For this review, take the finished solid that the model builds, in its own axes (mm). A direction names the side the tool comes from. Round coordinates to 2 decimals unless told otherwise and drop trailing zeros. Write each loop counter-clockwise with the first axis right and the second up, starting at its lowest first coordinate (ties: lowest second). Pieces come first, ordered by that corner, then holes. Notation, with made-up numbers: M 69,51.5 L 123,51.5 A31 ccw 123,81.5 Z; hole C -14,24.5 d2. An arc over 180 degrees is marked long. One line per question, with ' | ' between items.
```python
from build123d import *

# Parameters (mm, degrees)
F1_DEPTH  = 18.9992
F2_START  = -41.3258
F2_DEPTH  = 18.9992
F3_DEPTH  = 60.325
F4_DEPTH  = 60.325
F5_START  = -19.05
F5_DEPTH  = 41.275
F6_DEPTH  = 25.4
F7_R      = 3.302
F8_R      = 7.874
F9_R      = 6.35
F10_DEPTH = 22.353


with BuildPart() as f1:
    # F0 (on Front) → F1 (new body)
    with BuildSketch(Plane.XZ):
        with BuildLine():
            ThreePointArc((-171.8564, 22.352), (-210.0136507731, 38.1572507731), (-194.2084, 0))
            Line((-194.2084, 0), (-194.2084, 9.652))
            ThreePointArc((-194.2084, 9.652), (-203.1886561211, 31.3322561211), (-181.5084, 22.352))
            Line((-181.5084, 22.352), (-171.8564, 22.352))
        make_face()
        with BuildLine():
            Line((-194.2084, 9.652), (-194.2084, 0))
            ThreePointArc((-194.2084, 0), (-178.4031492269, 6.5467492269), (-171.8564, 22.352))
            Line((-171.8564, 22.352), (-181.5084, 22.352))
            ThreePointArc((-181.5084, 22.352), (-185.2281438789, 13.3717438789), (-194.2084, 9.652))
        make_face()
        with BuildLine():
            Line((-194.2084, 0), (-149.7584, 0))
            Line((-149.7584, 0), (-166.2684, 22.352))
            Line((-166.2684, 22.352), (-171.8564, 22.352))
            ThreePointArc((-171.8564, 22.352), (-178.4031492269, 6.5467492269), (-194.2084, 0))
        make_face()
        Polygon((-149.7584, 0), (-102.362, 0), (-108.3564, 22.352), (-166.2684, 22.352), align=None)
    extrude(amount=-F1_DEPTH)



with BuildPart() as f2:
    # F0 (on Front) → F2 (new body)
    with BuildSketch(Plane.XZ.offset(F2_START)):
        with BuildLine():
            ThreePointArc((-171.8564, 22.352), (-210.0136507731, 38.1572507731), (-194.2084, 0))
            Line((-194.2084, 0), (-194.2084, 9.652))
            ThreePointArc((-194.2084, 9.652), (-203.1886561211, 31.3322561211), (-181.5084, 22.352))
            Line((-181.5084, 22.352), (-171.8564, 22.352))
        make_face()
        with BuildLine():
            Line((-194.2084, 0), (-149.7584, 0))
            Line((-149.7584, 0), (-166.2684, 22.352))
            Line((-166.2684, 22.352), (-171.8564, 22.352))
            ThreePointArc((-171.8564, 22.352), (-178.4031492269, 6.5467492269), (-194.2084, 0))
        make_face()
        with BuildLine():
            Line((-194.2084, 9.652), (-194.2084, 0))
            ThreePointArc((-194.2084, 0), (-178.4031492269, 6.5467492269), (-171.8564, 22.352))
            Line((-171.8564, 22.352), (-181.5084, 22.352))
            ThreePointArc((-181.5084, 22.352), (-185.2281438789, 13.3717438789), (-194.2084, 9.652))
        make_face()
        Polygon((-149.7584, 0), (-102.362, 0), (-108.3564, 22.352), (-166.2684, 22.352), align=None)
    extrude(amount=-F2_DEPTH)


with BuildPart() as f1_1:
    add(f1.part)

    add(f2.part)  # F3 merges F2
    # F0 (on Front) → F3 (join, through all)
    with BuildSketch(Plane.XZ):
        Polygon((-149.7584, 0), (-102.362, 0), (-108.3564, 22.352), (-166.2684, 22.352), align=None)
    extrude(amount=-F3_DEPTH)



with BuildPart() as f4:
    # F0 (on Front) → F4 (new body)
    with BuildSketch(Plane.XZ):
        Polygon((-76.962, 0), (0, 0), (0, 22.352), (-44.1198, 22.352), (-76.962, 22.352), align=None)
    extrude(amount=-F4_DEPTH)


with BuildPart() as f1_2:
    add(f1_1.part)

    add(f4.part)  # F5 merges F4
    # F0 (on Front) → F5 (join)
    with BuildSketch(Plane.XZ.offset(F5_START)):
        Polygon((-102.362, 0), (-76.962, 0), (-76.962, 22.352), (-108.3564, 22.352), align=None)
    extrude(amount=-F5_DEPTH)

    # F0 (on Front) → F6 (join)
    with BuildSketch(Plane.XZ):
        with BuildLine():
            ThreePointArc((-63.1698, 57.15), (-66.7439846384, 38.4343576341), (-76.962, 22.352))
            Line((-76.962, 22.352), (-44.1198, 22.352))
            Line((-44.1198, 22.352), (-44.1198, 52.07))
            ThreePointArc((-44.1198, 52.07), (-45.6076975516, 55.6621024484), (-49.1998, 57.15))
            Line((-49.1998, 57.15), (-63.1698, 57.15))
        make_face()
    extrude(amount=-F6_DEPTH)

    # F7
    f7_edges = [f1_2.edges().sort_by_distance(p)[0] for p in [
        (-44.1198, 12.7, 22.352),
        (-171.8564, 9.4996, 22.352),
        (-171.8564, 50.8254, 22.352),
    ]]
    fillet(f7_edges, radius=F7_R)

    # F8
    f8_edges = [f1_2.edges().sort_by_distance(p)[0] for p in [
        (0, 30.1625, 22.352),
    ]]
    fillet(f8_edges, radius=F8_R)

    # F9 (on face) → F10 (cut, through all)
    with BuildSketch(Plane.XY.offset(22.352)):
        with Locations((-38.862, 37.973)):
            Circle(F9_R)
    extrude(amount=-F10_DEPTH, mode=Mode.SUBTRACT)


solid = f1_2.part
```
Item 1: Mouldability with a two-part tool opening along Y and no side actions: class faces 5 (the face through (-93, 19.05, 11)), 6 (the face through (-56, 13, 57.15)), 7 (the face through (-158.129, 30.006, 11.332)) as +Y half, -Y half, draft (parallel to the pull), parting line (faces both ways), or undercut.
Results:
face 5: -Y half | face 6: draft | face 7: undercut
Item 2: Take a section at A-A (y = 16). Write out the cut boundary in (x, z), then the cut area to 3 significant figures.
Results:
outline: M -194.21,0 L -102.36,0 L -108.36,22.35 L -168.77,22.35 A3.3 cw -172.04,25.23 A22.35 ccw long Z; M -76.96,0 L 0,0 L 0,14.48 A7.87 ccw -7.87,22.35 L -40.82,22.35 A3.3 cw -44.12,25.65 L -44.12,52.07 A5.08 ccw -49.2,57.15 L -63.17,57.15 A50.8 cw -76.96,22.35 Z; hole C -194.21,22.35 d25.4 | area: 5,180 mm2
Item 3: To check wall thickness, follow line 1 along X through (y, z) = (14.5, 13); line 2 along X through (y, z) = (16, 17.5); line 3 along Y through (x, z) = (-179, 33.5) (3 decimals). State the ranges of each line that lie inside material, in increasing order. Write a range as from..to.
Results:
line 1: -214.51..-202.8, -185.62..-105.85, -76.96..0 | line 2: -216.03..-205.95, -182.47..-107.06, -76.96..-0.6 | line 3: 0..18.999, 41.326..60.325
Item 4: Take a section at B-B (x = -198). Write out the cut boundary in (y, z) (3 decimals).
Results:
outline: M 0,0.324 L 18.999,0.324 L 18.999,10.231 L 0,10.231 Z; M 0,34.473 L 18.999,34.473 L 18.999,44.38 L 0,44.38 Z; M 41.326,0.324 L 60.325,0.324 L 60.325,10.231 L 41.326,10.231 Z; M 41.326,34.473 L 60.325,34.473 L 60.325,44.38 L 41.326,44.38 Z
Item 5: Insertion check: pin 1 Ø5.5 at (y, z) = (5, 7) entering from -X; pin 2 Ø3 at (y, z) = (10.5, 43.5) entering from +X; pin 3 Ø20.5 at (x, z) = (-194.21, 22.35) entering from -Y; pin 4 Ø8 at (y, z) = (49.5, 27.5) entering from +X. Each pin has a flat end and moves straight along its axis. Give the tip position at first contact, or say it passes through.
Results:
pin 1: x = -212.67 | pin 2: x = -44.12 | pin 3: through | pin 4: x = -171.27
Item 6: Take a section at D-D (z = 38). Write out the cut boundary in (x, y) (3 decimals), then the cut area to 3 significant figures.
Results:
outline: M -210.169,0 L -178.247,0 L -178.247,18.999 L -210.169,18.999 Z; M -210.169,41.326 L -178.247,41.326 L -178.247,60.325 L -210.169,60.325 Z; M -66.918,0 L -44.12,0 L -44.12,25.4 L -66.918,25.4 Z | area: 1,790 mm2
Item 7: Machinability: for faces 1 (the face through (-105.317, 9.392, 11.02)), 2 (the face through (-66.646, 12.522, 38.684)), 3 (the face through (-87, 36, 22.352)), 4 (the face through (-76.962, 9, 11)), which of the approach directions +Z, -Z, +X, -X, +Y, -Y give a long, thin tool a straight path to every point of the face, cutting with its end or side? Answer none if there is none.
Results:
face 1: +Z, -Y | face 2: +Z, +Y, -Y | face 3: +Z, +Y | face 4: +Z, -Z, -Y
Item 8: Take a section at C-C (z = 28.5). Write out the cut boundary in (x, y) (3 decimals), then the cut area to 3 significant figures.
Results:
outline: M -215.698,0 L -205.321,0 L -205.321,18.999 L -215.698,18.999 Z; M -215.698,41.326 L -205.321,41.326 L -205.321,60.325 L -215.698,60.325 Z; M -183.096,0 L -172.719,0 L -172.719,18.999 L -183.096,18.999 Z; M -183.096,41.326 L -172.719,41.326 L -172.719,60.325 L -183.096,60.325 Z; M -72.021,0 L -44.12,0 L -44.12,25.4 L -72.021,25.4 Z | area: 1,500 mm2
